```python
from build123d import *

# Parameters (mm, degrees)
BOX_W        = 10
BOX_H        = 17
BOX_DEPTH    = 14
BOX001_W     = 10
BOX001_H     = 10
BOX001_DEPTH = 10


with BuildPart() as box:
    # Box → Box (new body)
    with BuildSketch(Plane.XY):
        with Locations((5, 8.5)):
            Rectangle(BOX_W, BOX_H)
    extrude(amount=BOX_DEPTH)


with BuildPart() as fusion:
    # Box001 → Box001 (new body)
    with BuildSketch(Plane(origin=(10, 0, 0), x_dir=(1, 0, 0), z_dir=(0, 0, 1))):
        with Locations((5, 5)):
            Rectangle(BOX001_W, BOX001_H)
    extrude(amount=BOX001_DEPTH)

    # Fusion: union Box
    add(box.part)


solid = fusion.part
```
The listing builds one solid part. Answer for the finished solid, in the listing's coordinates (mm). A direction names the side the tool comes from. Coordinates: 2 decimals unless noted, no trailing zeros. Write each loop counter-clockwise with the first axis right and the second up, starting at its lowest first coordinate (ties: lowest second). Pieces come first, ordered by that corner, then holes. Notation, with made-up numbers: (20, 78.5) - (69, 78.5) arc R19 ccw to (69, 98.5) - close; hole circle Ø2 at (40.5, 88). An arc over 180 degrees is marked (long way). Return JSON: item names as keys, results as strings. Group by question number.
Q1. The part is cut by section B-B on y = 3.5. Write down the section's boundary in (x, z), and give its area (3 significant figures).
Q2. Flat-ended cylindrical pins translate along their axes: pin 1 Ø3 at (x, z) = (14.5, 11) entering from +Y; pin 2 Ø3 at (x, y) = (13, 4) entering from +Z. Find the tip coordinate at first contact, or state that the pin passes through.
Q3. Which of the six approach directions +Z, -Z, +X, -X, +Y, -Y give full straight-line access (tool end or side, diameter ignored) to faces 1 (the flat face through (15, 5, 10)), 2 (the flat face through (15, 10, 5)), 3 (the flat face through (5, 17, 7))?
Q4. The part is cut by section C-C on x = 18.75. Write down the section's boundary in (y, z), and give its area (3 significant figures).
Q5. Find the intervals of material crossed by line 1 along Z through (x, y) = (12, 4.5), in increasing order. Write a range as [from, to].
Q6. The part is cut by section A-A on z = 1.25. Write down the section's boundary in (x, y).
Q7. The part is cut by section D-D on z = 12.5. Write down the section's boundary in (x, y).
Evaluation:
{
 "1": {"outline": "(0, 0) - (20, 0) - (20, 10) - (10, 10) - (10, 14) - (0, 14) - close", "area": "240 mm2"},
 "2": {"pin 1": "stops at y = 10", "pin 2": "stops at z = 10"},
 "3": {"face 1": "+Z, +X, +Y, -Y", "face 2": "+Z, -Z, +X, +Y", "face 3": "+Z, -Z, +X, -X, +Y"},
 "4": {"outline": "(0, 0) - (10, 0) - (10, 10) - (0, 10) - close", "area": "100 mm2"},
 "5": {"line 1": "z = [0, 10]"},
 "6": {"outline": "(0, 0) - (20, 0) - (20, 10) - (10, 10) - (10, 17) - (0, 17) - close"},
 "7": {"outline": "(0, 0) - (10, 0) - (10, 17) - (0, 17) - close"}
}
